Design review of the part built by this model. Coordinates are the model's own, in mm. Face numbers are marked on the shaded views. A direction names the side the tool comes from. Coordinates: 2 decimals unless noted, no trailing zeros. Loops run counter-clockwise (first coordinate to the right, second up) from the corner with the lowest first, then second, coordinate; pieces in that order, holes last.
from build123d import *

# Parameters (mm, degrees)
SKETCH1_R           = 1.85
BOSS_EXTRUDE1_DEPTH = 3.1
SKETCH2_R           = 1.5
BOSS_EXTRUDE2_DEPTH = 1
SKETCH3_R           = 1.1
BOSS_EXTRUDE3_DEPTH = 2
SKETCH6_W           = 5
SKETCH6_H           = 5
BOSS_EXTRUDE4_DEPTH = 30
SKETCH7_R           = 1
CUT_EXTRUDE1_DEPTH  = 24


with BuildPart() as part:
    # Sketch1 → Boss-Extrude1 (new body)
    with BuildSketch(Plane(origin=(0, 0, 0), x_dir=(1, 0, 0), z_dir=(0, 1, 0))):
        with Locations(Location((0, 0, 0), (0, 0, 90))):
            Circle(SKETCH1_R)
    extrude(amount=BOSS_EXTRUDE1_DEPTH)

    # Sketch2 → Boss-Extrude2 (add)
    with BuildSketch(Plane(origin=(0, 3.1, 0), x_dir=(1, 0, 0), z_dir=(0, 1, 0))):
        with Locations(Location((0, 0, 0), (0, 0, 270))):
            Circle(SKETCH2_R)
    extrude(amount=BOSS_EXTRUDE2_DEPTH)

    # Sketch3 → Boss-Extrude3 (add)
    with BuildSketch(Plane(origin=(0, 4.1, 0), x_dir=(1, 0, 0), z_dir=(0, 1, 0))):
        with Locations(Location((0, 0, 0), (0, 0, 270))):
            Circle(SKETCH3_R)
    extrude(amount=BOSS_EXTRUDE3_DEPTH)

    # Loft1: read off the stored shape, not the designer's step
    # Loft1: loft between two sections, ruled curve by curve
    loft1_from = [
        Edge.make_bspline([(0, 6.1, 1.85), (3.7, 6.1, 1.85), (3.7, 6.1, -1.85), (0, 6.1, -1.85), (-3.7, 6.1, -1.85), (-3.7, 6.1, 1.85), (0, 6.1, 1.85)], [0, 0, 0, 0, 0.5, 0.5, 0.5, 1, 1, 1, 1], 3, [1, 0.333333333, 0.333333333, 1, 0.333333333, 0.333333333, 1]),
    ]
    loft1_to = [
        Edge.make_bspline([(0.620465421, 8.6, 0.968257539), (2.556980499, 8.6, -0.272673303), (1.316049657, 8.6, -2.209188381), (-0.620465421, 8.6, -0.968257539), (-2.556980499, 8.6, 0.272673303), (-1.316049657, 8.6, 2.209188381), (0.620465421, 8.6, 0.968257539)], [0, 0, 0, 0, 0.5, 0.5, 0.5, 1, 1, 1, 1], 3, [1, 0.333333333, 0.333333333, 1, 0.333333333, 0.333333333, 1]),
    ]
    loft1 = Solid(Shell([*[Face.make_surface_from_curves(loft1_from[k], loft1_to[k]) for k in range(1)], Face(Wire(loft1_from)), Face(Wire(loft1_to))]))
    add(loft1)

    # Sketch6 → Boss-Extrude4 (add)
    with BuildSketch(Plane.XZ):
        Rectangle(SKETCH6_W, SKETCH6_H)
    extrude(amount=BOSS_EXTRUDE4_DEPTH)

    # Sketch7 → Cut-Extrude1 (cut)
    with BuildSketch(Plane.XZ.offset(30)):
        with Locations(Location((0, 0, 0), (0, 0, 270))):
            Circle(SKETCH7_R)
    extrude(amount=-CUT_EXTRUDE1_DEPTH, mode=Mode.SUBTRACT)


solid = part.part
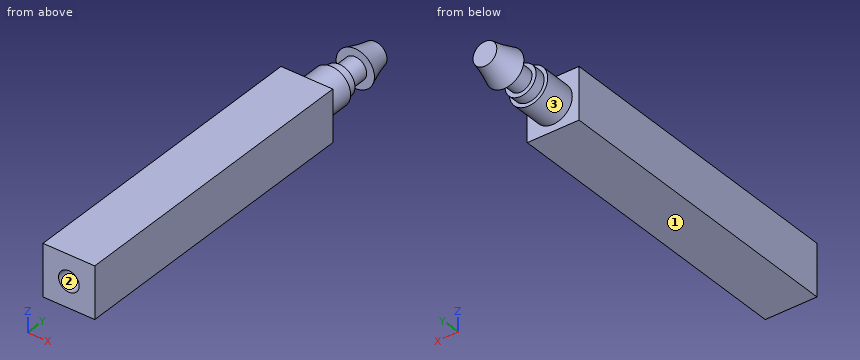
Q1. For line 1 (X direction, y = -14.75, z = 0); line 2 (Z direction, x = -0.1, y = -21); line 3 (Y direction, x = 1.25, z = 2.35), list the stretches that pass through material, from the lowest coordinate up.
Q2. Take a section at B-B, the plane y = 3.5. Write out the cut boundary in (x, z).
Q3. Clearance check with a flat-ended pin moving along its axis: pin 1 Ø0.6 at (x, z) = (0, -0.5) entering from -Y. State where the tip first meets the part, or that it passes through.
Q4. Machinability: for the marked faces 1, 2 and 3, which of the approach directions +Z, -Z, +X, -X, +Y, -Y give a long, thin tool a straight path to every point of the face, cutting with its end or side? Answer none if there is none.
Q5. Take a section at A-A, the plane y = -15. Write out the cut boundary in (x, z).
Entries:
1. line 1: x = -2.5 to -1, 1 to 2.5
1. line 2: z = -2.5 to -0.99, 0.99 to 2.5
1. line 3: y = -30 to 0
2. outline: circle Ø3 at (0, 0)
3. pin 1: stops at y = -6
4. face 1: -Z, +X, -X, +Y, -Y
4. face 2: -Y
4. face 3: +Y
5. outline: (-2.5, -2.5) - (2.5, -2.5) - (2.5, 2.5) - (-2.5, 2.5) - close; hole circle Ø2 at (0, 0)
